```python
from build123d import *

# Parameters (mm, degrees)
BOSS_EXTRUDE1_DEPTH = 12
CUT_EXTRUDE1_DEPTH  = 9.75
CUT_EXTRUDE4_START  = -4.4
CUT_EXTRUDE4_DEPTH  = 2.8
SKETCH3_R           = 1.45
CUT_EXTRUDE2_DEPTH  = 18
BOSS_EXTRUDE2_DEPTH = 29
SKETCH5_R           = 1.95
SKETCH5_R_2         = 2.6
CUT_EXTRUDE3_DEPTH  = 14.5
BOSS_EXTRUDE3_DEPTH = 2
BOSS_EXTRUDE4_START = -22
BOSS_EXTRUDE4_DEPTH = 2
CUT_EXTRUDE5_DEPTH  = 5.2
SKETCH9_W           = 30
SKETCH9_H           = 12
CUT_EXTRUDE6_DEPTH  = 0.5


with BuildPart() as part:
    # Sketch1 → Boss-Extrude1 (new body)
    with BuildSketch(Plane.XY):
        with BuildLine():
            Line((-5.280588843, 25), (-5.280588843, 41))
            Line((-5.280588843, 41), (5.219411157, 41))
            Line((5.219411157, 41), (5.219411157, 37.5))
            ThreePointArc((5.219411157, 37.5), (9.719411157, 33), (14.219411157, 37.5))
            Line((14.219411157, 37.5), (14.219411157, 41))
            Line((14.219411157, 41), (24.719411157, 41))
            Line((24.719411157, 41), (24.719411157, 25))
            Line((24.719411157, 25), (12.269411157, 25))
            Line((12.269411157, 25), (12.269411157, 26.8))
            Line((12.269411157, 26.8), (7.169411157, 26.8))
            Line((7.169411157, 26.8), (7.169411157, 25))
            Line((7.169411157, 25), (-5.280588843, 25))
        make_face()
    extrude(amount=-BOSS_EXTRUDE1_DEPTH)

    # Sketch2 → Cut-Extrude1 (cut)
    with BuildSketch(Plane.XY):
        with BuildLine():
            Line((4.369411157, 37.5), (4.369411157, 41))
            Line((4.369411157, 41), (15.069411157, 41))
            Line((15.069411157, 41), (15.069411157, 37.5))
            ThreePointArc((15.069411157, 37.5), (9.719411157, 32.15), (4.369411157, 37.5))
        make_face()
    extrude(amount=-CUT_EXTRUDE1_DEPTH, mode=Mode.SUBTRACT)

    # Sketch7 → Cut-Extrude4 (cut)
    with BuildSketch(Plane.XY.offset(CUT_EXTRUDE4_START)):
        with BuildLine():
            Line((3.244411157, 37.5), (3.244411157, 41))
            Line((3.244411157, 41), (16.194411157, 41))
            Line((16.194411157, 41), (16.194411157, 37.5))
            ThreePointArc((16.194411157, 37.5), (9.719411157, 31.025), (3.244411157, 37.5))
        make_face()
    extrude(amount=-CUT_EXTRUDE4_DEPTH, mode=Mode.SUBTRACT)

    # Sketch3 → Cut-Extrude2 (cut)
    with BuildSketch(Plane(origin=(0, 41, 0), x_dir=(1, 0, 0), z_dir=(0, 1, 0))):
        with Locations((20.219411157, 6)):
            Circle(SKETCH3_R)
        with Locations((-0.780588843, 6)):
            Circle(SKETCH3_R)
    extrude(amount=-CUT_EXTRUDE2_DEPTH, mode=Mode.SUBTRACT)

    # Sketch4 → Boss-Extrude2 (add)
    with BuildSketch(Plane.XY):
        Polygon((-1.280588843, 25), (-1.280588843, 29), (20.719411157, 29), (20.719411157, 25), (12.269411157, 25), (12.269411157, 26.8), (7.169411157, 26.8), (7.169411157, 25), align=None)
    extrude(amount=BOSS_EXTRUDE2_DEPTH)

    # Sketch5 → Cut-Extrude3 (cut, symmetric)
    with BuildSketch(Plane(origin=(0, 29, 0), x_dir=(1, 0, 0), z_dir=(0, 1, 0))):
        with Locations((9.719411157, -21)):
            Circle(SKETCH5_R)
        with Locations((9.719411157, -8)):
            Circle(SKETCH5_R)
        with Locations((9.719411157, 5)):
            Circle(SKETCH5_R_2)
    extrude(amount=CUT_EXTRUDE3_DEPTH, both=True, mode=Mode.SUBTRACT)

    # Sketch6 → Boss-Extrude3 (add)
    with BuildSketch(Plane.ZY.offset(1.280588843)):
        Polygon((29, 29), (0, 41), (0, 29), align=None)
    extrude(amount=-BOSS_EXTRUDE3_DEPTH)

    # Sketch6<2> → Boss-Extrude4 (add)
    with BuildSketch(Plane.ZY.offset(1.280588843).offset(BOSS_EXTRUDE4_START)):
        Polygon((29, 29), (0, 41), (0, 29), align=None)
    extrude(amount=BOSS_EXTRUDE4_DEPTH)

    # Sketch8 → Cut-Extrude5 (cut)
    with BuildSketch(Plane.XY):
        with BuildLine():
            Line((3.719411157, 37.5), (3.719411157, 41))
            Line((3.719411157, 41), (15.719411157, 41))
            Line((15.719411157, 41), (15.719411157, 37.5))
            ThreePointArc((15.719411157, 37.5), (9.719411157, 31.5), (3.719411157, 37.5))
        make_face()
    extrude(amount=-CUT_EXTRUDE5_DEPTH, mode=Mode.SUBTRACT)

    # Sketch9 → Cut-Extrude6 (cut)
    with BuildSketch(Plane(origin=(0, 41, 0), x_dir=(1, 0, 0), z_dir=(0, 1, 0))):
        with Locations((9.719411157, 6)):
            Rectangle(SKETCH9_W, SKETCH9_H)
    extrude(amount=-CUT_EXTRUDE6_DEPTH, mode=Mode.SUBTRACT)


solid = part.part
```
Part model, mm, in its own coordinate system. A direction names the side the tool comes from. Round coordinates to 2 decimals unless told otherwise and drop trailing zeros. Write each loop counter-clockwise with the first axis right and the second up, starting at its lowest first coordinate (ties: lowest second). Pieces come first, ordered by that corner, then holes. Notation, with made-up numbers: M -12.5,59 L 42.5,59 A23 ccw 42.5,73 Z; hole C -20,59 d1. An arc over 180 degrees is marked long. One line per question, with ' | ' between items.
(1) Saw through at C-C on z = -5. Write the cut outline in (x, y) (3 decimals).
Answer key:
outline: M -5.281,25 L -1.831,25 L -1.831,40.5 L -5.281,40.5 Z; M 0.269,25 L 7.119,25 L 7.119,31.57 A6.475 cw 3.244,37.5 L 3.244,40.5 L 0.269,40.5 Z; M 12.319,25 L 19.169,25 L 19.169,40.5 L 16.194,40.5 L 16.194,37.5 A6.475 cw 12.319,31.57 Z; M 21.269,25 L 24.719,25 L 24.719,40.5 L 21.269,40.5 Z
(2) Saw through at B-B on y = 27.25. Write the cut outline in (x, z).
Answer key:
outline: M -5.28,-12 L 24.72,-12 L 24.72,0 L 20.72,0 L 20.72,29 L -1.28,29 L -1.28,0 L -5.28,0 Z; hole C -0.78,-6 d2.9; hole C 9.72,-5 d5.2; hole C 9.72,8 d3.9; hole C 9.72,21 d3.9; hole C 20.22,-6 d2.9
(3) Saw through at D-D on z = 22.5. Write the cut outline in (x, y).
Answer key:
outline: M -1.28,25 L 7.17,25 L 7.17,26.8 L 8.47,26.8 L 8.47,29 L 0.72,29 L 0.72,31.69 L -1.28,31.69 Z; M 10.97,26.8 L 12.27,26.8 L 12.27,25 L 20.72,25 L 20.72,31.69 L 18.72,31.69 L 18.72,29 L 10.97,29 Z
(4) Two-plate mould, pull along Z, no slides. Class faces 5 (the face through (15, 35.5, -7.2)), 6 (the face through (-5.281, 33, -6)), 7 (the face through (15.5, 35.4, -4.4)), 8 (the face through (19.733, 34.916, 14.703)): released by +Z, released by -Z, zero draft, split by the parting line, or undercut.
Answer key:
face 5: undercut | face 6: zero draft | face 7: undercut | face 8: released by +Z
(5) Saw through at A-A on y = 40. Count the separate pieces of the cut face and the enclosed holes in it, then the cut area to 3 significant figures.
Answer key:
separate pieces: 2 | enclosed holes: 2 | area: 220 mm^2
(6) Pin check, flat tips, straight feed: pin 1 (1.5 mm diameter, centred on x = 13, y = 37.5, fed in from +Z); pin 2 (1.2 mm diameter, centred on x = -4, y = 31, fed in from +Z); pin 3 (3.5 mm diameter, centred on y = 37, z = 12.5, fed in from +X); pin 4 (9 mm diameter, centred on x = 10.5, z = 12.5, fed in from +Y). Stop position of each tip, or through.
Answer key:
pin 1: passes through | pin 2: stops at z = 0 | pin 3: stops at x = 20.72 | pin 4: stops at y = 29
(7) Probe line 1 along X through (y, z) = (25.75, 18.5); line 2 along X through (y, z) = (31.5, 2.5); line 3 along X through (y, z) = (30.25, -6). List the from-to ranges inside material, lowest first.
Answer key:
line 1: x = -1.28 to 7.17, 12.27 to 20.72 | line 2: x = -1.28 to 0.72, 18.72 to 20.72 | line 3: x = -5.28 to -2.23, 0.67 to 7.32, 12.12 to 18.77, 21.67 to 24.72
(8) 3-axis set-ups, long thin cutter, end or side, ignore diameter. For faces 1 (the face through (12.269, 26, 12)), 2 (the face through (-1.281, 31, 11)), 3 (the face through (14.219, 39, -11)), 4 (the face through (0.719, 32, 8)): which of +Z, -Z, +X, -X, +Y, -Y reach the whole face in a straight line?
Answer key:
face 1: +Z, -Z, -Y | face 2: +Z, -X, +Y, -Y | face 3: +Z, -Z, +Y | face 4: +Z, +Y
